```python
from build123d import *

# Parameters (mm, degrees)
SKETCH_1_R          = 25
EXTRUDE_1_DEPTH     = 7
SKETCH_2_R          = 10
EXTRUDE_2_DEPTH     = 30
FILLET_1_R          = 3
SKETCH_3_R          = 4
CUT_EXTRUDE_3_DEPTH = 52.176166328


with BuildPart() as part:
    # Эскиз1 → Вытянуть1 (new body)
    with BuildSketch(Plane.XY):
        Circle(SKETCH_1_R)
    extrude(amount=EXTRUDE_1_DEPTH)

    # Эскиз2 → Вытянуть2 (add)
    with BuildSketch(Plane.XY.offset(7)):
        Circle(SKETCH_2_R)
    extrude(amount=EXTRUDE_2_DEPTH)

    # Скругление1
    fillet_1_edges = [part.edges().sort_by_distance(p)[0] for p in [
        (-10, 0, 7),
    ]]
    fillet(fillet_1_edges, radius=FILLET_1_R)

    # Эскиз3 → Вытянуть3 (cut, through all)
    with BuildSketch(Plane.XY.offset(37)):
        Circle(SKETCH_3_R)
    extrude(amount=-CUT_EXTRUDE_3_DEPTH, mode=Mode.SUBTRACT)


solid = part.part
```
Geometry: final body of the model. Coordinates: model frame, mm. A direction names the side the tool comes from. Round coordinates to 2 decimals unless told otherwise and drop trailing zeros. Write each loop counter-clockwise with the first axis right and the second up, starting at its lowest first coordinate (ties: lowest second). Pieces come first, ordered by that corner, then holes. Notation, with made-up numbers: M -17.5,81 L 5.5,81 A24 ccw 5.5,106 Z; hole C 6.5,-10 d11. An arc over 180 degrees is marked long. Answer in a Markdown table with one row per item. Add a question column.
(1) Cut plane C-C, the plane z = 13.5. Return the cut outline in (x, y).
(2) Reachability of faces 4 (the face through (11, -11, 7)), 5 (the face through (23.846, 7.509, 3.451)) from +Z, -Z, +X, -X, +Y, -Y: full face, straight path, thin tool, end or side. Return the list, or none.
(3) Cut plane D-D, the plane y = 19. Return the cut outline in (x, z), then the cut area to 3 significant figures.
(4) Draft query along Y for faces 1 (the face through (-2.17, -9.76, 23.31)), 2 (the face through (-0.867, -3.905, 18.759)), 3 (the face through (0, -5, 0)). Return one class per face: pulls with the +Y half, pulls with the -Y half, needs draft (parallel to the pull), parting line crosses it, or undercut.
(5) Cut plane A-A, the plane y = 0. Return the cut outline in (x, z), then the cut area to 3 significant figures.
(6) Ray query, L1, parallel to Y at x = 0, z = 24; L2, parallel to Z at x = 17, y = 1.5; L3, parallel to Y at x = -1, z = 12. Return the intervals inside material, ascending.
(7) Contact query for flat-ended pins moving along their axis: pin 1 (8 mm diameter, centred on x = -11.5, z = 29, fed in from -Y); pin 2 (12 mm diameter, centred on x = -4.5, y = -20, fed in from +Z); pin 3 (5 mm diameter, centred on x = 12, y = -12.5, fed in from -Z); pin 4 (10 mm diameter, centred on x = 10, z = 13.5, fed in from -Y). Output: stop coordinate, or through.
Established:
| question | item | result |
|---|---|---|
| 1 | outline | C 0,0 d20; hole C 0,0 d8 |
| 2 | face 4 | +Z |
| 2 | face 5 | +Z, -Z |
| 3 | outline | M -16.25,0 L 16.25,0 L 16.25,7 L -16.25,7 Z |
| 3 | area | 227 mm² |
| 4 | face 1 | parting line crosses it |
| 4 | face 2 | undercut |
| 4 | face 3 | needs draft |
| 5 | outline | M -25,0 L -4,0 L -4,37 L -10,37 L -10,10 A3 cw -13,7 L -25,7 Z; M 4,0 L 25,0 L 25,7 L 13,7 A3 cw 10,10 L 10,37 L 4,37 Z |
| 5 | area | 658 mm² |
| 6 | L1 | -10 to -4, 4 to 10 |
| 6 | L2 | 0 to 7 |
| 6 | L3 | -9.95 to -3.87, 3.87 to 9.95 |
| 7 | pin 1 | y = -6.61 |
| 7 | pin 2 | z = 7 |
| 7 | pin 3 | z = 0 |
| 7 | pin 4 | y = -8.66 |
